The listing builds one solid part. Answer for the finished solid, in the listing's coordinates (mm). Give positions to 0.01 mm unless a question says otherwise; leave off trailing zeros. Write each loop counter-clockwise with the first axis right and the second up, starting at its lowest first coordinate (ties: lowest second). Pieces come first, ordered by that corner, then holes. Notation, with made-up numbers: M -36,64 L 22,64 A21 cw 22,79 Z; hole C 2,55.5 d3. An arc over 180 degrees is marked long. Answer as a JSON object with one key per item and string values.
```python
from build123d import *

# Parameters (mm, degrees)
SALIENTE_EXTRUIR1_DEPTH = 3.2
CORTAR_EXTRUIR1_DEPTH   = 3.2
REDONDEO1_R             = 3
CROQUIS3_R              = 2.05
CROQUIS3_R_2            = 1.55
CORTAR_EXTRUIR2_DEPTH   = 3.2
CROQUIS4_R              = 1.55
CORTAR_EXTRUIR3_DEPTH   = 3.2


with BuildPart() as part:
    # Croquis1 → Saliente-Extruir1 (new body)
    with BuildSketch(Plane(origin=(0, 0, 0), x_dir=(1, 0, 0), z_dir=(0, 1, 0))):
        Polygon((7, 66.1), (10, 66.1), (10, 62.9), (7, 62.9), (7, 61.5), (3, 61.5), (3, 62.9), (0, 62.9), (0, 57), (-3, 57), (-3, 51), (0, 51), (0, 0), (165, 0), (165, 1.5), (168, 1.5), (168, 7.5), (165, 7.5), (165, 13.4), (162, 13.4), (162, 12), (158, 12), (158, 13.4), (155, 13.4), (155, 16.6), (158, 16.6), (158, 18), (162, 18), (162, 16.6), (165, 16.6), (165, 22.5), (168, 22.5), (168, 28.5), (165, 28.5), (165, 370), (30, 370), (30, 366.9), (21.6, 366.9), (21.6, 363.9), (23, 363.9), (23, 359.9), (21.6, 359.9), (21.6, 356.9), (18.4, 356.9), (18.4, 359.9), (17, 359.9), (17, 363.9), (18.4, 363.9), (18.4, 366.9), (10, 366.9), (10, 370), (0, 370), (0, 358), (-3, 358), (-3, 352), (0, 352), (0, 346.1), (3, 346.1), (3, 347.5), (7, 347.5), (7, 346.1), (10, 346.1), (10, 342.9), (7, 342.9), (7, 341.5), (3, 341.5), (3, 342.9), (0, 342.9), (0, 337), (-3, 337), (-3, 331), (0, 331), (0, 218), (-3, 218), (-3, 212), (0, 212), (0, 206.1), (3, 206.1), (3, 207.5), (7, 207.5), (7, 206.1), (10, 206.1), (10, 202.9), (7, 202.9), (7, 201.5), (3, 201.5), (3, 202.9), (0, 202.9), (0, 197), (-3, 197), (-3, 191), (0, 191), (0, 78), (-3, 78), (-3, 72), (0, 72), (0, 66.1), (3, 66.1), (3, 67.5), (7, 67.5), align=None)
    extrude(amount=SALIENTE_EXTRUIR1_DEPTH)

    # Croquis2 → Cortar-Extruir1 (cut)
    with BuildSketch(Plane.XZ):
        with BuildLine():
            Line((165, -370), (33, -370))
            ThreePointArc((33, -370), (69.526447022, -189.023572292), (165, -31))
            Line((165, -31), (165, -370))
        make_face()
    extrude(amount=-CORTAR_EXTRUIR1_DEPTH, mode=Mode.SUBTRACT)

    # Redondeo1
    redondeo1_edges = [part.edges().sort_by_distance(p)[0] for p in [
        (33, 1.6, -370),
    ]]
    fillet(redondeo1_edges, radius=REDONDEO1_R)

    # Croquis3 → Cortar-Extruir2 (cut)
    with BuildSketch(Plane(origin=(0, 3.2, 0), x_dir=(1, 0, 0), z_dir=(0, 1, 0))):
        with Locations((40, 80)):
            Circle(CROQUIS3_R)
        with Locations((90, 80)):
            Circle(CROQUIS3_R)
        with Locations((40, 230)):
            Circle(CROQUIS3_R)
        with Locations((20, 95)):
            Circle(CROQUIS3_R_2)
        with Locations((20, 215)):
            Circle(CROQUIS3_R_2)
        with Locations((100, 95)):
            Circle(CROQUIS3_R_2)
        with Locations((25, 65)):
            Circle(CROQUIS3_R_2)
        with Locations((25, 190)):
            Circle(CROQUIS3_R_2)
        with Locations((110, 65)):
            Circle(CROQUIS3_R_2)
    extrude(amount=-CORTAR_EXTRUIR2_DEPTH, mode=Mode.SUBTRACT)

    # Croquis4 → Cortar-Extruir3 (cut)
    with BuildSketch(Plane.XZ):
        with Locations((15, -35)):
            Circle(CROQUIS4_R)
        with Locations((91, -35)):
            Circle(CROQUIS4_R)
        with Locations((15, -137)):
            Circle(CROQUIS4_R)
        with Locations((15, -170)):
            Circle(CROQUIS4_R)
        with Locations((33, -35)):
            Circle(CROQUIS4_R)
        with Locations((81.26, -35)):
            Circle(CROQUIS4_R)
        with Locations((33, -117.55)):
            Circle(CROQUIS4_R)
        with Locations((81.26, -109.93)):
            Circle(CROQUIS4_R)
        with Locations((28, -35)):
            Circle(CROQUIS4_R)
        with Locations((95.48, -35)):
            Circle(CROQUIS4_R)
        with Locations((28, -162.61)):
            Circle(CROQUIS4_R)
        with Locations((63.61, -162.61)):
            Circle(CROQUIS4_R)
        with Locations((117, -35)):
            Circle(CROQUIS4_R)
        with Locations((15, -111)):
            Circle(CROQUIS4_R)
        with BuildLine():
            Line((143, -30.5), (129, -30.5))
            ThreePointArc((129, -30.5), (127.585786438, -31.085786438), (127, -32.5))
            Line((127, -32.5), (127, -36.5))
            ThreePointArc((127, -36.5), (127.585786438, -37.914213562), (129, -38.5))
            Line((129, -38.5), (143, -38.5))
            ThreePointArc((143, -38.5), (144.414213562, -37.914213562), (145, -36.5))
            Line((145, -36.5), (145, -32.5))
            ThreePointArc((145, -32.5), (144.414213562, -31.085786438), (143, -30.5))
        make_face()
    extrude(amount=-CORTAR_EXTRUIR3_DEPTH, mode=Mode.SUBTRACT)


solid = part.part
```
1. A cutting plane is placed at A-A, the plane x = 132.5. Give the vertices of the cut face in (y, z).
Verdict:
{"outline": "M 0,-72.29 L 3.2,-72.29 L 3.2,-38.5 L 0,-38.5 Z; M 0,-30.5 L 3.2,-30.5 L 3.2,0 L 0,0 Z"}
2. Flat-ended cylindrical pins translate along their axes: pin 1 (1 mm diameter, centred on x = 20, y = 2, fed in from -Z); pin 2 (1.6 mm diameter, centred on y = 2, z = -68, fed in from -X); pin 3 (1 mm diameter, centred on x = 12.5, y = 1, fed in from -Z). Find the tip coordinate at first contact, or state that the pin passes through.
Verdict:
{"pin 1": "stops at z = -356.9", "pin 2": "stops at x = 0", "pin 3": "stops at z = -366.9"}
3. Consider line 1 along Z through (x, y) = (15, 2.45); line 2 along Z through (x, y) = (4, 1.15); line 3 along Z through (x, y) = (25, 1.05). Determine where each line is inside the solid, lowest interval first.
Verdict:
{"line 1": "z = -366.9 to -171.55, -168.45 to -138.55, -135.45 to -112.55, -109.45 to -36.55, -33.45 to 0", "line 2": "z = -370 to -347.5, -341.5 to -207.5, -201.5 to -67.5, -61.5 to 0", "line 3": "z = -366.9 to -191.55, -188.45 to -66.55, -63.45 to 0"}
4. A cutting plane is placed at D-D, the plane z = -261. Give the vertices of the cut face in (x, y), plus the area to 3 significant figures.
Verdict:
{"outline": "M 0,0 L 47.16,0 L 47.16,3.2 L 0,3.2 Z", "area": "151 mm2"}
5. A cutting plane is placed at C-C, the plane z = -322. Give the vertices of the cut face in (x, y), plus the area to 3 significant figures.
Verdict:
{"outline": "M 0,0 L 36.45,0 L 36.45,3.2 L 0,3.2 Z", "area": "117 mm2"}
6. A cutting plane is placed at B-B, the plane y = 2.3. Count the separate pieces of the cut face and the enclosed holes in it, plus the area to 3 significant figures.
Verdict:
{"separate pieces": "1", "enclosed holes": "24", "area": "30,500 mm2"}
